Source: CAD feature listing. Evaluate the final solid. Frame: model axes, mm. A direction names the side the tool comes from. Give positions to 0.01 mm unless a question says otherwise; leave off trailing zeros. Order: outer loops, then holes, each group sorted by start corner. A loop starts at its lowest first (then second) coordinate and runs counter-clockwise, first axis right, second up.
1) Section C-C, the plane z = -13. Return loops of the section in (x, y).
2) Material intervals for line 1 (Z direction, x = -1.5, y = 6.55); line 2 (Y direction, x = -6.5, z = -20.5), sorted ascending.
3) Section B-B, the plane x = -17. Return loops of the section in (y, z).
4) Section A-A, the plane y = 9.05. Return loops of the section in (x, z), plus the area to 3 significant figures.
5) Access query for faces 4 (the face through (0, 11, -20)), 5 (the face through (-12, 8, -31)). Directions: +Z, -Z, +X, -X, +Y, -Y. A direction counts if a zero-diameter tool reaches every point of the face in a straight line with its end or side. Return the directions, or none.
6) First-contact query: P1, Ø6, axis at x = -13, z = -13, coming from the -Y side. Flat tip, straight axial feed; report the tip coordinate or a pass-through.
7) Draft query along Z for faces 1 (the face through (-12, 9.95, -20)), 2 (the face through (-12, 9, 0)), 3 (the face through (-13, 5.75, -35)). Return one class per face: released by +Z, released by -Z, zero draft, split by the parting line, or undercut.
Autodesk Inventor part; units mm, degrees
ref_plane "YZ Plane" through (0, 0, 0) normal (1, 0, 0) x (0, 1, 0)
ref_plane "XZ Plane" through (0, 0, 0) normal (0, 1, 0) x (-1, 0, 0)
ref_plane "XY Plane" through (0, 0, 0) normal (0, 0, 1) x (1, 0, 0)
sketch "Sketch1" plane through (0, 0, 0) normal (0, 1, 0) x (-1, 0, 0)
  line L0 (0, 0) -> (25, 0)
  line L1 (25, 0) -> (25, -39)
  line L2 (25, -39) -> (0, -39)
  line L3 (0, -39) -> (0, 0)
  line L4 (0, -8) -> (25, -8)
  line L5 (25, -8) -> (25, -31)
  line L6 (25, -31) -> (0, -31)
  line L7 (0, -31) -> (0, -8)
  dimension "d0" = 39
  dimension "d1" = 25
  dimension "d2" = 23
  dimension "d3" = 8
  dimension "d4" = 8
extrude "Extrusion1" add sketch "Sketch1" along normal blind 11.5
sketch "Sketch3" plane through (0, 0, 0) normal (1, 0, 0) x (0, 0, -1)
  line L0 (0, 0) -> (0, 11.5)
  line L1 (0, 0) -> (39, 0)
  line L2 (8, 1.55) -> (31, 1.55)
  line L3 (31, 1.55) -> (31, 9.95)
  line L4 (31, 9.95) -> (8, 9.95)
  line L5 (8, 9.95) -> (8, 1.55)
  line L6 (8, 1.55) -> (31, 9.95) construction
  line L7 (31, 1.55) -> (8, 9.95) construction
  point P0 (0, 5.75)
  point P1 (19.5, 0)
  point P2 (19.5, 5.75)
  dimension "d9" = 23
  dimension "d10" = 8.4
  dimension "d25" = 8
extrude "Extrusion2" cut sketch "Sketch3" against normal through all
sketch "Sketch4" plane through (0, 0, 0) normal (1, 0, 0) x (0, 0, -1)
  line L0 (0, 0) -> (0, 11.5)
  line L1 (0, 5.75) -> (39, 5.75)
  line L2 (39, 0) -> (39, 11.5)
split body "Split1" sketch "Sketch4" result one side removed curves L1 removed pieces at (-8.3333, 0.5, -13)
properties part number "Servo mount top v2"
From the geometry:
1. outline: (-25, 9.95) - (0, 9.95) - (0, 11.5) - (-25, 11.5) - close
2. line 1: z = -39 to -31, -8 to 0
2. line 2: y = 9.95 to 11.5
3. outline: (5.75, -39) - (11.5, -39) - (11.5, 0) - (5.75, 0) - (5.75, -8) - (9.95, -8) - (9.95, -31) - (5.75, -31) - close
4. outline: (-25, -39) - (0, -39) - (0, -31) - (-25, -31) - close; (-25, -8) - (0, -8) - (0, 0) - (-25, 0) - close
4. area: 400 mm2
5. face 4: +Z, -Z, +X, +Y, -Y
5. face 5: +X, -X, -Y
6. P1: stops at y = 9.95
7. face 1: undercut
7. face 2: released by +Z
7. face 3: zero draft
